from build123d import *

# Parameters (mm, degrees)
SKETCH2_R           = 76
BOSS_EXTRUDE1_DEPTH = 15
SKETCH4_R           = 86
SKETCH4_R_2         = 76
BOSS_EXTRUDE2_DEPTH = 25
CUT_EXTRUDE1_DEPTH  = 10


with BuildPart() as part:
    # Sketch2 → Boss-Extrude1 (new body)
    with BuildSketch(Plane(origin=(0, 0, 0), x_dir=(1, 0, 0), z_dir=(0, 1, 0))):
        with Locations(Location((0, 0, 0), (0, 0, 270))):
            Circle(SKETCH2_R)
    extrude(amount=BOSS_EXTRUDE1_DEPTH)

    # Sketch4 → Boss-Extrude2 (add)
    with BuildSketch(Plane(origin=(0, 0, 0), x_dir=(-1, 0, 0), z_dir=(0, -1, 0))):
        with Locations(Location((0, 0, 0), (0, 0, 90))):
            Circle(SKETCH4_R)
        with Locations(Location((0, 0, 0), (0, 0, 90))):
            Circle(SKETCH4_R_2, mode=Mode.SUBTRACT)
    extrude(amount=-BOSS_EXTRUDE2_DEPTH)

    # Sketch5 → Cut-Extrude1 (cut)
    with BuildSketch(Plane(origin=(0, 25, 0), x_dir=(1, 0, 0), z_dir=(0, 1, 0))):
        Polygon((86, 0), (86, 2.38), (75.161889678, 2.38), (75.161889678, -2.38), (86.243553227, -2.38), align=None)
        Polygon((-86, 0), (-86, 2.38), (-75.22208349, 2.38), (-75.22208349, -2.38), (-86.457059311, -2.38), align=None)
        Polygon((0, 86), (2.38, 86), (2.38, 74.13986027), (-2.38, 74.13986027), (-2.38, 86.447056085), align=None)
        Polygon((0, -86), (2.38, -86), (2.38, -74.817551039), (-2.38, -74.817551039), (-2.38, -87.761718776), align=None)
    extrude(amount=-CUT_EXTRUDE1_DEPTH, mode=Mode.SUBTRACT)


solid = part.part
Design review of the part built by this model. Coordinates are the model's own, in mm. A direction names the side the tool comes from. Coordinates: 2 decimals unless noted, no trailing zeros. Order: outer loops, then holes, each group sorted by start corner. A loop starts at its lowest first (then second) coordinate and runs counter-clockwise, first axis right, second up.
Item 1: Take a section at B-B, the plane x = -8.5. Write out the cut boundary in (y, z), then the cut area to 3 significant figures.
Item 2: For line 1 (Y direction, x = 4.5, z = -67.5); line 2 (Z direction, x = -34, y = 24.25); line 3 (X direction, y = 17.75, z = 66.5), list the stretches that pass through material, from the lowest coordinate up.
Item 3: For faces 1 (the flat face through (-81, 20, -2.38)), 2 (the flat face through (2.38, 20, 81)), 3 (the cylindrical face through (-53.17, 19.93, 54.304)), 4 (the flat face through (57, 25, -56)), list the 3-axis set-ups (+Z, -Z, +X, -X, +Y, -Y) from which the entire face can be reached by the end or side of a thin tool; tool diameter is ignored.
Item 4: Take a section at C-C, the plane y = 4.5. Write out the cut boundary in (x, z).
Item 5: The part is to be moulded in two halves that separate along X. For faces 5 (the flat face through (51, 25, 57)), 6 (the cylindrical face through (-54.304, 19.93, -53.17)), 7 (the cylindrical face through (58.12, 12.32, 63.39)), say which applies: pulls with the +X half, pulls with the -X half, needs draft (parallel to the pull), parting line crosses it, or undercut.
Item 6: For pin 1 Ø1 at (x, z) = (-20, 2.5) entering from +Y; pin 2 Ø8 at (y, z) = (22.5, 79.5) entering from -X; pin 3 Ø10 at (x, y) = (41.5, 15) entering from +Z, all flat-tipped, find the tip position at first contact; note any pin that passes through.
Item 7: Take a section at D-D, the plane z = 0. Write out the cut boundary in (x, y), then the cut area to 3 significant figures.
Item 8: Take a section at A-A, the plane z = -23.5. Write out the cut boundary in (x, y).
The answers:
1. outline: (0, -85.58) - (25, -85.58) - (25, -75.52) - (15, -75.52) - (15, 75.52) - (25, 75.52) - (25, 85.58) - (0, 85.58) - close
1. area: 2,770 mm2
2. line 1: y = 0 to 15
2. line 2: z = -78.99 to -67.97, 67.97 to 78.99
2. line 3: x = -54.53 to -36.79, 36.79 to 54.53
3. face 1: +X, -X, +Y
3. face 2: +Z, -Z, +Y
3. face 3: +Y
3. face 4: +Z, -Z, +X, -X, +Y
4. outline: circle Ø172 at (0, 0)
5. face 5: needs draft
5. face 6: undercut
5. face 7: parting line crosses it
6. pin 1: stops at y = 15
6. pin 2: stops at x = -41.18
6. pin 3: stops at z = 77.87
7. outline: (-86, 0) - (86, 0) - (86, 15) - (-86, 15) - close
7. area: 2,580 mm2
8. outline: (-82.73, 0) - (82.73, 0) - (82.73, 25) - (72.28, 25) - (72.28, 15) - (-72.28, 15) - (-72.28, 25) - (-82.73, 25) - close
